Check sheet for the modelled part. Datum: model origin and axes. Units: mm. A direction names the side the tool comes from. Give positions to 0.01 mm unless a question says otherwise; leave off trailing zeros. Loops run counter-clockwise (first coordinate to the right, second up) from the corner with the lowest first, then second, coordinate; pieces in that order, holes last. Notation, with made-up numbers: (40.5, 7.25) - (92.5, 7.25) arc R19 cw to (92.5, 29.25) - close; hole circle Ø11 at (-8, 71). An arc over 180 degrees is marked (long way). Answer in a Markdown table with one row per item. Add a question column.
(1) Draft check along X on faces 3 (the face through (20.765, -39.923, 27.329)), 4 (the face through (-18, 18, 6.2)), 5 (the face through (-14.4, 7.4, 0)). Enter one of: released by +X, released by -X, zero draft, split by the parting line, or undercut.
(2) Set-up check for faces 1 (the face through (18, 18, 6.2)), 2 (the face through (-1, 1, 48.75)): record each of +Z, -Z, +X, -X, +Y, -Y from which the full face is reachable in a straight line by a thin tool's end or side.
(3) Thickness scan on L1, parallel to Y at x = 0, z = 2.75; L2, parallel to Z at x = 37, y = -2; L3, parallel to Z at x = 6, y = 1. Record the ranges inside material, lowest first.
(4) Sectioned sample at C-C on z = 3. Enter the section's corners in (x, y).
(5) Sectioned sample at A-A on y = 0. Enter the section's corners in (x, z), then the cut area to 3 significant figures.
(6) Go/stop test with flat-tipped pins: P1, Ø3, axis at x = 19.5, z = 25.5, coming from the -Y side; P2, Ø1.5, axis at x = 18, y = 16.5, coming from the -Z side; P3, Ø8, axis at x = -35.5, z = 18, coming from the -Y side. Record where each tip stops, or that it passes through.
(7) Sectioned sample at D-D on z = 39. Enter the section's corners in (x, y).
from build123d import *

# Parameters (mm, degrees)
SKETCH1_R           = 45
BOSS_EXTRUDE1_DEPTH = 48.75
SKETCH1_3_R         = 45
SKETCH1_3_R_2       = 31.5
CUT_EXTRUDE1_DEPTH  = 6.5
SKETCH1_4_R         = 15.75
SKETCH1_4_R_2       = 2.5
CUT_EXTRUDE2_DEPTH  = 6.2


with BuildPart() as part:
    # Sketch1 → Boss-Extrude1 (new body)
    with BuildSketch(Plane.XY):
        Circle(SKETCH1_R)
    extrude(amount=BOSS_EXTRUDE1_DEPTH)

    # Sketch1_3 → Cut-Extrude1 (cut)
    with BuildSketch(Plane.XY):
        Circle(SKETCH1_3_R)
        with Locations(Location((0, 0, 0), (0, 0, 180))):
            Circle(SKETCH1_3_R_2, mode=Mode.SUBTRACT)
    extrude(amount=CUT_EXTRUDE1_DEPTH, mode=Mode.SUBTRACT)

    # Sketch1_4 → Cut-Extrude2 (cut)
    with BuildSketch(Plane.XY):
        with Locations(Location((0, 0, 0), (0, 0, 180))):
            Circle(SKETCH1_4_R)
        with Locations(Location((-17.67766953, 17.67766953, 0), (0, 0, 180))):
            Circle(SKETCH1_4_R_2)
        with Locations(Location((17.67766953, 17.67766953, 0), (0, 0, 180))):
            Circle(SKETCH1_4_R_2)
        with Locations(Location((17.67766953, -17.67766953, 0), (0, 0, 180))):
            Circle(SKETCH1_4_R_2)
        with Locations(Location((-17.67766953, -17.67766953, 0), (0, 0, 180))):
            Circle(SKETCH1_4_R_2)
    extrude(amount=CUT_EXTRUDE2_DEPTH, mode=Mode.SUBTRACT)


solid = part.part
Reply:
| question | item | result |
|---|---|---|
| 1 | face 3 | split by the parting line |
| 1 | face 4 | undercut |
| 1 | face 5 | zero draft |
| 2 | face 1 | -Z |
| 2 | face 2 | +Z, +X, -X, +Y, -Y |
| 3 | L1 | -31.5 to -15.75, 15.75 to 31.5 |
| 3 | L2 | 6.5 to 48.75 |
| 3 | L3 | 6.2 to 48.75 |
| 4 | outline | circle Ø63 at (0, 0); hole circle Ø5 at (-17.68, -17.68); hole circle Ø5 at (-17.68, 17.68); hole circle Ø31.5 at (0, 0); hole circle Ø5 at (17.68, -17.68); hole circle Ø5 at (17.68, 17.68) |
| 5 | outline | (-45, 6.5) - (-31.5, 6.5) - (-31.5, 0) - (-15.75, 0) - (-15.75, 6.2) - (15.75, 6.2) - (15.75, 0) - (31.5, 0) - (31.5, 6.5) - (45, 6.5) - (45, 48.75) - (-45, 48.75) - close |
| 5 | area | 4,020 mm^2 |
| 6 | P1 | y = -41.24 |
| 6 | P2 | z = 6.2 |
| 6 | P3 | y = -32.14 |
| 7 | outline | circle Ø90 at (0, 0) |
